from build123d import *

# Parameters (mm, degrees)
ESQUISSE1_W                  = 0.6
ESQUISSE1_H                  = 0.6
BOSS_EXTRU_1_DEPTH           = 2.8
BOSS_EXTRU_1_DEPTH_BACK      = 1.1
ESQUISSE2_W                  = 0.6
ESQUISSE2_H                  = 0.575
ENL_V_MAT_EXTRU_1_DEPTH      = 1
ESQUISSE3_W                  = 0.6
ESQUISSE3_H                  = 0.6
BOSS_EXTRU_2_DEPTH           = 4
BOSS_EXTRU_2_DEPTH_BACK      = 4
ESQUISSE4_R                  = 0.674645205
ESQUISSE4_R_2                = 0.5
BOSS_EXTRU_3_DEPTH           = 0.01
ESQUISSE6_W                  = 0.6
ESQUISSE6_H                  = 0.6
ESQUISSE5_W                  = 0.6
ESQUISSE5_H                  = 0.6
ENL_V_MAT_EXTRU_2_DEPTH      = 0.1
ENL_V_MAT_EXTRU_2_DEPTH_BACK = 0.1
CHANFREIN1_SIZE              = 0.2


with BuildPart() as part:
    # Esquisse1 → Boss.-Extru.1 (new body, two sides)
    with BuildSketch(Plane.XY) as boss_extru_1_sk:
        Polygon((-0.675, 0.875), (-0.875, 0.675), (-0.875, -0.675), (-0.675, -0.875), (0.675, -0.875), (0.875, -0.675), (0.875, 0.675), (0.675, 0.875), align=None)
        Rectangle(ESQUISSE1_W, ESQUISSE1_H, mode=Mode.SUBTRACT)
    extrude(amount=BOSS_EXTRU_1_DEPTH)
    extrude(boss_extru_1_sk.sketch, amount=-BOSS_EXTRU_1_DEPTH_BACK)

    # Esquisse2 → Enl_v. mat.-Extru.1 (cut)
    with BuildSketch(Plane.XY.offset(2.8)):
        with Locations((0, -0.5875)):
            Rectangle(ESQUISSE2_W, ESQUISSE2_H)
    extrude(amount=-ENL_V_MAT_EXTRU_1_DEPTH, mode=Mode.SUBTRACT)

    # Esquisse3 → Boss.-Extru.2 (add, two sides)
    with BuildSketch(Plane.XY.offset(2.8)) as boss_extru_2_sk:
        Rectangle(ESQUISSE3_W, ESQUISSE3_H)
    extrude(amount=BOSS_EXTRU_2_DEPTH)
    extrude(boss_extru_2_sk.sketch, amount=-BOSS_EXTRU_2_DEPTH_BACK)

    # Esquisse4 → Boss.-Extru.3 (add)
    with BuildSketch(Plane.XY.offset(2.8)):
        Circle(ESQUISSE4_R)
        Circle(ESQUISSE4_R_2, mode=Mode.SUBTRACT)
    extrude(amount=BOSS_EXTRU_3_DEPTH)

    # Balayage1: sweep along a path in Esquisse25
    with BuildLine(Plane(origin=(0, 0, 0), x_dir=(0, 0, -1), z_dir=(1, 0, 0))) as balayage1_path:
        Line((2.565105715, 6), (2.565105715, 1.192347565))
        ThreePointArc((2.565105715, 1.192347565), (2.153394049, 0.286090658), (1.2, 0))
    # Esquisse6 → Balayage1 (sweep)
    with BuildSketch(Plane(origin=(0, 0, -1.2), x_dir=(-1, 0, 0), z_dir=(0, 0, -1))):
        Rectangle(ESQUISSE6_W, ESQUISSE6_H)
    sweep(path=balayage1_path.line)

    # Esquisse5 → Enl_v. mat.-Extru.2 (cut, two sides)
    with BuildSketch(Plane(origin=(0, 6, 0), x_dir=(1, 0, 0), z_dir=(0, 1, 0))) as enl_v_mat_extru_2_sk:
        with Locations((0, 2.565105715)):
            Rectangle(ESQUISSE5_W, ESQUISSE5_H)
    extrude(amount=ENL_V_MAT_EXTRU_2_DEPTH, mode=Mode.SUBTRACT)
    extrude(enl_v_mat_extru_2_sk.sketch, amount=-ENL_V_MAT_EXTRU_2_DEPTH_BACK, mode=Mode.SUBTRACT)

    # Chanfrein1
    chanfrein1_edges = [part.edges().sort_by_distance(p)[0] for p in [
        (-0.3, 5.9, -2.565105715),
        (0.3, 5.9, -2.565105715),
        (0, 5.9, -2.267831149),
        (0, 5.9, -2.862380281),
        (0.3, 0, 6.8),
        (0, 0.3, 6.8),
        (-0.3, 0, 6.8),
        (0, -0.3, 6.8),
    ]]
    chamfer(chanfrein1_edges, length=CHANFREIN1_SIZE)


solid = part.part
Read the model definition and answer for the solid it produces. Units are mm, in the model's axes. A direction names the side the tool comes from. Coordinates: 2 decimals unless noted, no trailing zeros. Loops run counter-clockwise (first coordinate to the right, second up) from the corner with the lowest first, then second, coordinate; pieces in that order, holes last.
Q1. Each of these flat-tipped pins is pushed along its axis until it touches: pin 1 Ø0.6 at (x, y) = (0, -0.5) entering from +Z; pin 2 Ø1.9 at (y, z) = (2, -2.5) entering from +X; pin 3 Ø1.9 at (y, z) = (3.5, -1.5) entering from -X. Where does it stop, or does it pass through?
Q2. The part is cut by section D-D on z = 3. Write down the section's boundary in (x, y), and give its area (3 significant figures).
Q3. Which of the six approach directions +Z, -Z, +X, -X, +Y, -Y give full straight-line access (tool end or side, diameter ignored) to faces 1 (the face through (0, 0.875, 1)), 2 (the face through (-0.3, 2.5, -2.5)), 3 (the face through (0.3, 2.3, -2.5))?
Q4. The part is cut by section C-C on y = 0. Write down the section's boundary in (x, z) (3 decimals).
Q5. The part is cut by section B-B on z = -1. Write down the section's boundary in (x, y) (3 decimals).
Q6. The part is cut by section A-A on x = 0. Write down the section's boundary in (y, z) (3 decimals).
Q7. Consider probe 1 along Y at (x, z) = (0.2, 3.25); probe 2 along Z at (x, y) = (-0.05, 5); probe 3 along Z at (x, y) = (-0.25, 0.75). Determine where each line is inside the solid, lowest interval first.
Results below:
1. pin 1: stops at z = 6.7
1. pin 2: stops at x = 0.3
1. pin 3: stops at x = -0.3
2. outline: (-0.3, -0.3) - (0.3, -0.3) - (0.3, 0.3) - (-0.3, 0.3) - close
2. area: 0.360 mm2
3. face 1: +Z, +X, -X, +Y
3. face 2: -Z, -X, +Y, -Y
3. face 3: -Z, +X, +Y, -Y
4. outline: (-0.875, -1.1) - (-0.3, -1.1) - (-0.3, -2.274) - (0.3, -2.274) - (0.3, -1.1) - (0.875, -1.1) - (0.875, 2.8) - (0.675, 2.8) - (0.675, 2.81) - (0.5, 2.81) - (0.5, 2.8) - (0.3, 2.8) - (0.3, 6.6) - (0.1, 6.8) - (-0.1, 6.8) - (-0.3, 6.6) - (-0.3, 2.8) - (-0.5, 2.8) - (-0.5, 2.81) - (-0.675, 2.81) - (-0.675, 2.8) - (-0.875, 2.8) - close
5. outline: (-0.875, -0.675) - (-0.675, -0.875) - (0.675, -0.875) - (0.875, -0.675) - (0.875, 0.675) - (0.675, 0.875) - (-0.675, 0.875) - (-0.875, 0.675) - close
6. outline: (-0.875, -1.1) - (-0.3, -1.1) - (-0.3, -1.2) arc R1.501 ccw to (1.233, -2.862) - (5.7, -2.862) - (5.9, -2.662) - (5.9, -2.468) - (5.7, -2.268) - (1.152, -2.268) arc R0.907 cw to (0.3, -1.2) - (0.3, -1.1) - (0.875, -1.1) - (0.875, 2.8) - (0.675, 2.8) - (0.675, 2.81) - (0.5, 2.81) - (0.5, 2.8) - (0.3, 2.8) - (0.3, 6.6) - (0.1, 6.8) - (-0.1, 6.8) - (-0.3, 6.6) - (-0.3, 1.8) - (-0.875, 1.8) - close; (-0.675, 2.8) - (-0.5, 2.8) - (-0.5, 2.81) - (-0.675, 2.81) - close
7. probe 1: y = -0.3 to 0.3
7. probe 2: z = -2.86 to -2.27
7. probe 3: z = -2.8 to -2.15, -1.1 to 2.8
